Could you check a few things on this model? Use its own coordinates, in mm. A direction names the side the tool comes from. Round coordinates to 2 decimals unless told otherwise and drop trailing zeros. Write each loop counter-clockwise with the first axis right and the second up, starting at its lowest first coordinate (ties: lowest second). Pieces come first, ordered by that corner, then holes. Notation, with made-up numbers: (-2.75, -1) - (17.25, -1) arc R15 ccw to (17.25, 8) - close; hole circle Ø11 at (86.5, -7.5). An arc over 180 degrees is marked (long way). Write each question's results on one line, items separated by ' | '. Start each with the question number.
(1) Please list where these lines run through material, in increasing order: line 1 (Z direction, x = 0, y = -1.8); line 2 (Z direction, x = 0, y = -2.75); line 3 (Z direction, x = 0, y = -8). Write a range as [from, to].
(2) Imagine slicing it at A-A on y = 14. Write out the boundary of the cut face in (x, z) (3 decimals).
(3) For P1, Ø2.5, axis at x = -2.55, z = -6.99, coming from the +Y side; P2, Ø16, axis at x = 0, z = 0, coming from the -Y side; P3, Ø1.1, axis at x = -7.33, z = 1.29, coming from the -Y side; P4, Ø3, axis at x = -12.5, y = -7.5, coming from the -Z side, each with a flat end and sliding along its axis, tell me the tip position at first contact or that it passes through.
(4) On a 3-axis mill with a long thin cutter (end or side, diameter ignored), from which of +Z, -Z, +X, -X, +Y, -Y can I reach the whole of each face in a straight line? I mean faces 1 (the cylindrical face through (-2.67, -2.32, -6.05)), 2 (the cylindrical face through (5.45, -5.2, 1.72)), 3 (the flat face through (0, -14.224, -12)). Say none if no direction works.
```python
from build123d import *

# Parameters (mm, degrees)
F0_R      = 19.05
F1_DEPTH  = 15.748
F3_R      = 8.8392
F4_DEPTH  = 11.176
F5_R      = 0.254
F6_R      = 0.9525
F7_DEPTH  = 25.4
F8_R      = 5.715
F9_DEPTH  = 1.27
F11_R     = 18.0989194231
F11_R_2   = 11.2988088197
F12_DEPTH = 14.224
F10_R     = 5.715
F13_DEPTH = 19.05
F14_T     = 3.175


# Not quite as in the source:
# - a feature of the source that left no trace in its solid (it failed there, or was rolled back) is left out
# - a shell that OpenCascade refuses in one call is made with other operations: the cavity is built on its own and cut out


with BuildPart() as f1:
    # F0 (on Front) → F1 (new body)
    with BuildSketch(Plane.XZ):
        Circle(F0_R)
    extrude(amount=F1_DEPTH)

    # F3 (on face) → F4 (cut)
    with BuildSketch(Plane.XZ.offset(15.748)):
        Circle(F3_R)
    extrude(amount=-F4_DEPTH, mode=Mode.SUBTRACT)

    # F5
    f5_edges = [f1.edges().sort_by_distance(p)[0] for p in [
        (-8.8392, -15.748, 0),
        (8.8392, -10.16, 0),
        (-8.8392, -4.572, 0),
        (-19.05, -15.748, 0),
    ]]
    fillet(f5_edges, radius=F5_R)

    # F6 (on face) → F7 (cut)
    with BuildSketch(Plane.XZ.offset(4.572)):
        with Locations((0, 7.4422)):
            Circle(F6_R)
        with Locations((4.7837539488, 5.7010559546)):
            Circle(F6_R)
        with Locations((7.3291362595, 1.2923244678)):
            Circle(F6_R)
        with Locations((6.44513426, -3.7211)):
            Circle(F6_R)
        with Locations((2.5453823107, -6.9933804224)):
            Circle(F6_R)
        with Locations((-2.5453823107, -6.9933804224)):
            Circle(F6_R)
        with Locations((-6.44513426, -3.7211)):
            Circle(F6_R)
        with Locations((-7.3291362595, 1.2923244678)):
            Circle(F6_R)
        with Locations((-4.7837539488, 5.7010559546)):
            Circle(F6_R)
    extrude(amount=-F7_DEPTH, mode=Mode.SUBTRACT)

    # F8 (on face) → F9 (join)
    with BuildSketch(Plane.XZ.offset(4.572)):
        Circle(F8_R)
    extrude(amount=F9_DEPTH)

    # F11 (on face) → F12 (cut)
    with BuildSketch(Plane(origin=(0, 0, 0), x_dir=(-1, 0, 0), z_dir=(0, 1, 0))):
        Circle(F11_R)
        Circle(F11_R_2, mode=Mode.SUBTRACT)
    extrude(amount=-F12_DEPTH, mode=Mode.SUBTRACT)

    # F10 (on face) → F13 (join)
    with BuildSketch(Plane(origin=(0, 0, 0), x_dir=(-1, 0, 0), z_dir=(0, 1, 0))):
        Circle(F10_R)
    extrude(amount=F13_DEPTH)

    # F14: shell of thickness 3.175, made by hand


with BuildPart() as f14_core1:
    # F14_t2: copy of F1
    add(f1.part)

    # the walls: a layer under each face that stays
    f14_faces = [f14_core1.faces().sort_by_distance(p)[0] for p in [
        (-19.05, -7.747, 0),
        (-17.78, 0, -5.08),
        (-12.5306666667, -15.748, -12.5306666667),
        (18.0989194231, -7.112, 0),
        (12.065946282, -14.224, -12.065946282),
        (-8.8392, -10.16, 0),
        (11.2988088197, -7.112, 0),
        (-8.7648051224, -4.6463948776, 0),
        (-7.5325392131, 0, -7.5325392131),
        (-5.7234666667, -4.572, -5.7234666667),
        (-3.4978823107, -2.286, -6.9933804224),
        (-7.39763426, -2.286, -3.7211),
        (1.5928823107, -2.286, -6.9933804224),
        (5.715, 9.525, 0),
        (5.49263426, -2.286, -3.7211),
        (-8.2816362595, -2.286, 1.2923244678),
        (-5.7362539488, -2.286, 5.7010559546),
        (-0.9525, -2.286, 7.4422),
        (6.3766362595, -2.286, 1.2923244678),
        (3.8312539488, -2.286, 5.7010559546),
        (-5.715, -5.207, 0),
        (0, -5.842, 0),
    ]]
    thicken(f14_faces, amount=-F14_T, mode=Mode.SUBTRACT)

    # F14_s3 → F14_t4 (revolve, cut)
    with BuildSketch(Plane.XY):
        Polygon((-18.0671694231, -14.19225), (-21.2739194231, -14.224), (-21.2739194231, -17.399), (-18.0989194231, -17.399), align=None)
    revolve(axis=Axis((0, -14.224, 0), (0, 1, 0)), mode=Mode.SUBTRACT)

    # F14_s5 → F14_t6 (revolve, cut)
    with BuildSketch(Plane.XY):
        Polygon((-11.3305588197, -14.19225), (-11.2988088197, -17.399), (-8.1238088197, -17.399), (-8.1238088197, -14.224), align=None)
    revolve(axis=Axis((0, -14.224, 0), (0, 1, 0)), mode=Mode.SUBTRACT)

    # F14_s7 → F14_t8 (revolve, cut)
    with BuildSketch(Plane.XY):
        Polygon((-5.74675, 0.03175), (-5.715, -3.175), (-2.54, -3.175), (-2.54, 0), align=None)
    revolve(axis=Axis((0, 0, 0), (0, 1, 0)), mode=Mode.SUBTRACT)

    # F14_s9 → F14_t10 (revolve, cut)
    with BuildSketch(Plane.XY):
        Polygon((5.74675, -4.60375), (5.715, -1.397), (2.54, -1.397), (2.54, -4.572), align=None)
    revolve(axis=Axis((0, -4.572, 0), (0, -1, 0)), mode=Mode.SUBTRACT)


with BuildPart() as f1_1:
    add(f1.part)

    # what is left inside the walls is the cavity
    f14_cavity = [f14_core1.part.solids().sort_by_distance(p)[0] for p in [
        (2.50825, 4.572, 0),
    ]]
    add(f14_cavity, mode=Mode.SUBTRACT)


solid = f1_1.part
```
Response:
1) line 1: [-19.05, -18.1], [-11.3, -2.54], [2.54, 6.49], [8.39, 11.3], [18.1, 19.05] | line 2: [-19.05, -18.1], [-11.3, 6.49], [8.39, 11.3], [18.1, 19.05] | line 3: [-19.05, -18.1], [-11.3, -8.84], [8.84, 11.3], [18.1, 19.05]
2) outline: circle Ø11.43 at (0, 0); hole circle Ø5.08 at (0, 0)
3) P1: y = 0 | P2: y = -5.84 | P3: through | P4: z = -15.55
4) face 1: +Y, -Y | face 2: -Y | face 3: +Y
